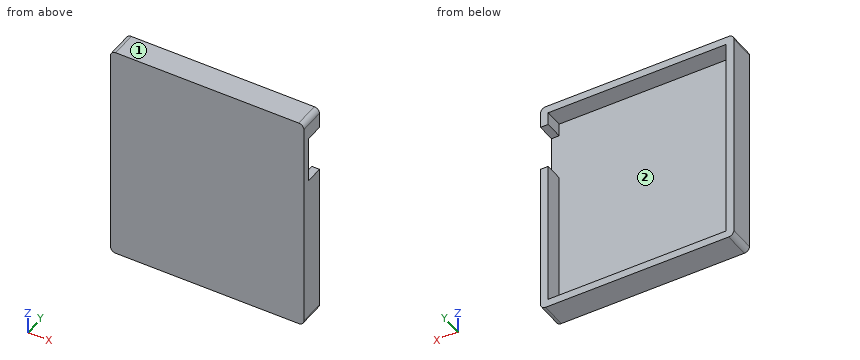
```python
from build123d import *

# Parameters (mm, degrees)
SKETCH1_W           = 75
SKETCH1_H           = 86
SKETCH1_W_2         = 69
SKETCH1_H_2         = 80
BOSS_EXTRUDE1_DEPTH = 3
SKETCH1_4_W         = 75
SKETCH1_4_H         = 86
SKETCH1_4_W_2       = 69
SKETCH1_4_H_2       = 80
BOSS_EXTRUDE2_DEPTH = 10
SKETCH2_W           = 18
SKETCH2_H           = 7
CUT_EXTRUDE1_DEPTH  = 10
FILLET1_R           = 2


with BuildPart() as part:
    # Sketch1 → Boss-Extrude1 (new body)
    # profile 1 of 2: a face of its own
    with BuildSketch(Plane(origin=(0, 0, 0), x_dir=(1, 0, 0), z_dir=(0, 1, 0))):
        Rectangle(SKETCH1_W, SKETCH1_H)
        Rectangle(SKETCH1_W_2, SKETCH1_H_2, mode=Mode.SUBTRACT)
    # profile 2 of 2: a face of its own
    with BuildSketch(Plane(origin=(0, 0, 0), x_dir=(1, 0, 0), z_dir=(0, 1, 0))):
        Rectangle(SKETCH1_W_2, SKETCH1_H_2)
    extrude(amount=BOSS_EXTRUDE1_DEPTH)

    # Sketch1_4 → Boss-Extrude2 (add)
    with BuildSketch(Plane(origin=(0, 0, 0), x_dir=(1, 0, 0), z_dir=(0, 1, 0))):
        Rectangle(SKETCH1_4_W, SKETCH1_4_H)
        Rectangle(SKETCH1_4_W_2, SKETCH1_4_H_2, mode=Mode.SUBTRACT)
    extrude(amount=BOSS_EXTRUDE2_DEPTH)

    # Sketch2 → Cut-Extrude1 (cut)
    with BuildSketch(Plane(origin=(37.5, 0, 0), x_dir=(0, 0, -1), z_dir=(1, 0, 0))):
        with Locations((-26, 6.5)):
            Rectangle(SKETCH2_W, SKETCH2_H)
    extrude(amount=-CUT_EXTRUDE1_DEPTH, mode=Mode.SUBTRACT)

    # Fillet1
    fillet1_edges = [part.edges().sort_by_distance(p)[0] for p in [
        (-37.5, 5, -43),
        (37.5, 5, -43),
        (37.5, 5, 43),
        (-37.5, 5, 43),
    ]]
    fillet(fillet1_edges, radius=FILLET1_R)


solid = part.part
```
Work out the finished part from the listing and answer in its coordinate system (mm). Face numbers are marked on the shaded views. Round coordinates to 2 decimals unless told otherwise and drop trailing zeros. Write each loop counter-clockwise with the first axis right and the second up, starting at its lowest first coordinate (ties: lowest second). Pieces come first, ordered by that corner, then holes. Notation, with made-up numbers: (50.25, 76.25) -> (101.25, 76.25) arc R24 cw to (101.25, 101.25) -> close; hole circle Ø11 at (40, -38.75). An arc over 180 degrees is marked (long way). Write each question's results on one line, items separated by ' | '.
1) The part is cut by section A-A (z = 9.5). Write down the section's boundary in (x, y), and give its area (3 significant figures).
Findings:
outline: (-37.5, 0) -> (37.5, 0) -> (37.5, 10) -> (34.5, 10) -> (34.5, 3) -> (-34.5, 3) -> (-34.5, 10) -> (-37.5, 10) -> close | area: 267 mm²
2) Flat-ended cylindrical pins translate along their axes: pin 1 (3 mm diameter, centred on x = 24, z = -4, fed in from +Y); pin 2 (0.9 mm diameter, centred on x = 36.5, y = 6, fed in from +Z). Find the tip coordinate at first contact, or state that the pin passes through.
Findings:
pin 1: stops at y = 3 | pin 2: stops at z = 42.92
3) The part is cut by section B-B (x = -29.5). Write down the section's boundary in (y, z).
Findings:
outline: (0, -43) -> (10, -43) -> (10, -40) -> (3, -40) -> (3, 40) -> (10, 40) -> (10, 43) -> (0, 43) -> close
4) The part is cut by section C-C (y = 8). Write down the section's boundary in (x, z).
Findings:
outline: (-37.5, -41) arc R2 ccw to (-35.5, -43) -> (35.5, -43) arc R2 ccw to (37.5, -41) -> (37.5, 17) -> (34.5, 17) -> (34.5, -40) -> (-34.5, -40) -> (-34.5, 40) -> (34.5, 40) -> (34.5, 35) -> (37.5, 35) -> (37.5, 41) arc R2 ccw to (35.5, 43) -> (-35.5, 43) arc R2 ccw to (-37.5, 41) -> close
5) The part is cut by section D-D (z = 28). Write down the section's boundary in (x, y), and give its area (3 significant figures).
Findings:
outline: (-37.5, 0) -> (37.5, 0) -> (37.5, 3) -> (-34.5, 3) -> (-34.5, 10) -> (-37.5, 10) -> close | area: 246 mm²
6) Consider line 1 along Z through (x, y) = (28, 6.75); line 2 along X through (y, z) = (4.25, -2); line 3 along Y through (x, z) = (33.5, 3). Determine where each line is inside the solid, lowest interval first. Write a range as [from, to].
Findings:
line 1: z = [-43, -40], [40, 43] | line 2: x = [-37.5, -34.5], [34.5, 37.5] | line 3: y = [0, 3]
7) For a pull along X with two mould halves and no side action, classify the marked faces 1 and 2 as +X half, -X half, draft (parallel to the pull), parting line (faces both ways), or undercut.
Findings:
face 1: draft | face 2: undercut
